For this review, take the finished solid that the model builds, in its own axes (mm). Give positions to 0.01 mm unless a question says otherwise; leave off trailing zeros. Write each loop counter-clockwise with the first axis right and the second up, starting at its lowest first coordinate (ties: lowest second). Pieces come first, ordered by that corner, then holes. Notation, with made-up numbers: M 15.25,53 L 50.25,53 A27 cw 50.25,71 Z; hole C 77,23 d3. An arc over 180 degrees is marked long. Write item = value, one per line.
```python
from build123d import *

# Parameters (mm, degrees)
SKETCH1_R           = 23.6982
SKETCH1_R_2         = 22.225
BOSS_EXTRUDE1_DEPTH = 450
CUT_EXTRUDE2_START  = -28.81672
SKETCH3_W           = 4.856446364
SKETCH3_H           = 19.05
CUT_EXTRUDE2_DEPTH  = 1.71492
CIRPATTERN4_COUNT   = 3


with BuildPart() as part:
    # Sketch1 → Boss-Extrude1 (new body)
    with BuildSketch(Plane.XY):
        Circle(SKETCH1_R)
        Circle(SKETCH1_R_2, mode=Mode.SUBTRACT)
    extrude(amount=BOSS_EXTRUDE1_DEPTH)

    # Sketch3 → Cut-Extrude2 (cut)
    with BuildSketch(Plane(origin=(0, 50.8, 0), x_dir=(1, 0, 0), z_dir=(0, 1, 0)).offset(CUT_EXTRUDE2_START)):
        with Locations((0.840723182, -434.125)):
            Rectangle(SKETCH3_W, SKETCH3_H)
    cut_extrude2 = extrude(amount=CUT_EXTRUDE2_DEPTH, mode=Mode.SUBTRACT)

    # CirPattern4: Cut-Extrude2 ×3 about axis
    cirpattern4_axis = Axis((0, 0, 0), (0, 0, 1))
    for i in range(1, CIRPATTERN4_COUNT):
        add(cut_extrude2.rotate(cirpattern4_axis, i * 360 / CIRPATTERN4_COUNT), mode=Mode.SUBTRACT)


solid = part.part
```
1. We need section B-B, the plane x = -9.5. Write out the cut boundary in (y, z).
Responses:
outline = M -21.71,0 L -20.09,0 L -20.09,450 L -21.71,450 Z; M 20.09,0 L 21.71,0 L 21.71,450 L 20.09,450 Z
2. For line 1 along Y through (x, z) = (0, 282) (3 decimals); line 2 along Y through (x, z) = (9.5, 175); line 3 along X through (y, z) = (8.5, 103), list the stretches that pass through material, from the lowest coordinate up. Write a range as from..to.
Responses:
line_1 = -23.698..-22.225, 22.225..23.698
line_2 = -21.71..-20.09, 20.09..21.71
line_3 = -22.12..-20.54, 20.54..22.12
3. We need section A-A, the plane y = 0. Write out the cut boundary in (x, z) (3 decimals).
Responses:
outline = M -23.698,0 L -22.225,0 L -22.225,450 L -23.698,450 Z; M 22.225,0 L 23.698,0 L 23.698,450 L 22.225,450 Z
4. The part is to be moulded in two halves that separate along X. For faces 1 (the face through (-5.137, -23.135, 221.85)), 2 (the face through (21.199, 6.676, 221.85)), say which applies: +X half, -X half, draft (parallel to the pull), parting line (faces both ways), or undercut.
Responses:
face_1 = parting line
face_2 = undercut
5. We need section C-C, the plane z = 343. Write out the cut boundary in (x, y) (3 decimals), then the cut area to 3 significant figures.
Responses:
outline = C 0,0 d47.396; hole C 0,0 d44.45
area = 213 mm2
6. Insertion check: P1, Ø4, axis at x = -12, y = 14.5, coming from the +Z side; P2, Ø1.5, axis at y = -13, z = 152.5, coming from the -X side; P3, Ø1.2, axis at y = 22.5, z = 430, coming from the +X side; P4, Ø1.6, axis at y = 22.5, z = 432, coming from the -X side. Each pin has a flat end and moves straight along its axis. Give the tip position at first contact, or say it passes through.
Responses:
P1 = through
P2 = -20.29
P3 = 9.06
P4 = -9.52
